For this review, take the finished solid that the model builds, in its own axes (mm). A direction names the side the tool comes from. Round coordinates to 2 decimals unless told otherwise and drop trailing zeros. Write each loop counter-clockwise with the first axis right and the second up, starting at its lowest first coordinate (ties: lowest second). Pieces come first, ordered by that corner, then holes. Notation, with made-up numbers: (26.5, -31.5) -> (81.5, -31.5) arc R20 ccw to (81.5, -21.5) -> close; hole circle Ø7 at (39.5, 58). An arc over 180 degrees is marked (long way). Answer in a Markdown table with one row per item.
from build123d import *

# Parameters (mm, degrees)
DODANIE_WYCI_GNI_CIE1_DEPTH = 130
SKORUPA1_T                  = -0.5
WYTNIJ_WYCI_GNI_CIE1_REACH  = 132
SZKIC2_W                    = 206
SZKIC2_H                    = 132
SZKIC4_R                    = 2
WYTNIJ_WYCI_GNI_CIE2_DEPTH  = 10
SZKIC5_R                    = 21.15
SZKIC5_R_2                  = 12.5
WYTNIJ_WYCI_GNI_CIE3_DEPTH  = 10
SZKIC6_R                    = 10
SZKIC6_R_2                  = 6
WYTNIJ_WYCI_GNI_CIE4_DEPTH  = 10
SZKIC7_R                    = 10.25
WYTNIJ_WYCI_GNI_CIE5_DEPTH  = 10


with BuildPart() as part:
    # Szkic1 → Dodanie-wyciągnięcie1 (new body)
    with BuildSketch(Plane.XY):
        Polygon((0, 403), (0, 185), (-30, 185), (-30, 0), (450, 0), (450, 403), align=None)
    extrude(amount=DODANIE_WYCI_GNI_CIE1_DEPTH)

    # Skorupa1
    skorupa1_openings = [part.faces().sort_by_distance(p)[0] for p in [
        (140, 196, 130),
    ]]
    offset(amount=SKORUPA1_T, openings=skorupa1_openings, kind=Kind.INTERSECTION)

    # Szkic2 → Wytnij-wyciągnięcie1 (cut, up to next)
    with BuildSketch(Plane(origin=(0, 0, 0), x_dir=(-1, 0, 0), z_dir=(0, 0, -1)), mode=Mode.PRIVATE) as wytnij_wyci_gni_cie1_sk1:
        with Locations((-329, 214)):
            Rectangle(SZKIC2_W, SZKIC2_H)
    wytnij_wyci_gni_cie1_tool1 = extrude(wytnij_wyci_gni_cie1_sk1.sketch, amount=-WYTNIJ_WYCI_GNI_CIE1_REACH, mode=Mode.PRIVATE) & part.part
    add(wytnij_wyci_gni_cie1_tool1.solids().sort_by_distance((329, 214, 0))[0], mode=Mode.SUBTRACT)

    # Szkic4 → Wytnij-wyciągnięcie2 (cut)
    with BuildSketch(Plane(origin=(0, 0, 0), x_dir=(-1, 0, 0), z_dir=(0, 0, -1))):
        with Locations((-114.4, 386.6)):
            Circle(SZKIC4_R)
        with Locations((-74.7, 365.2)):
            Circle(SZKIC4_R)
        with Locations((-74.7, 335.2)):
            Circle(SZKIC4_R)
        with Locations((-114.4, 356.6)):
            Circle(SZKIC4_R)
        with Locations((-74.7, 305.2)):
            Circle(SZKIC4_R)
        with Locations((-114.4, 326.6)):
            Circle(SZKIC4_R)
    extrude(amount=-WYTNIJ_WYCI_GNI_CIE2_DEPTH, mode=Mode.SUBTRACT)

    # Szkic5 → Wytnij-wyciągnięcie3 (cut)
    with BuildSketch(Plane(origin=(0, 403, 0), x_dir=(1, 0, 0), z_dir=(0, 1, 0))):
        with Locations((222.5, -77.9)):
            Circle(SZKIC5_R)
        with Locations((225.5, -23.7)):
            Circle(SZKIC5_R_2)
        with Locations((267.5, -23.7)):
            Circle(SZKIC5_R_2)
        with Locations((183.5, -23.7)):
            Circle(SZKIC5_R_2)
    extrude(amount=-WYTNIJ_WYCI_GNI_CIE3_DEPTH, mode=Mode.SUBTRACT)

    # Szkic6 → Wytnij-wyciągnięcie4 (cut)
    with BuildSketch(Plane.ZY.offset(30)):
        with Locations((74.5, 145)):
            Circle(SZKIC6_R)
        with Locations((74.5, 82)):
            Circle(SZKIC6_R)
        with Locations((13, 148)):
            Circle(SZKIC6_R_2)
        with Locations((13, 108)):
            Circle(SZKIC6_R_2)
        with Locations((13, 68)):
            Circle(SZKIC6_R_2)
    extrude(amount=-WYTNIJ_WYCI_GNI_CIE4_DEPTH, mode=Mode.SUBTRACT)

    # Szkic7 → Wytnij-wyciągnięcie5 (cut)
    with BuildSketch(Plane(origin=(0.5, 0, 0), x_dir=(0, 0, -1), z_dir=(1, 0, 0))):
        with Locations((-76, 224.23)):
            Circle(SZKIC7_R)
        with Locations((-76, 246.58)):
            Circle(SZKIC7_R)
        with BuildLine():
            Line((-87.5, 233.905), (-87.5, 236.905))
            ThreePointArc((-87.5, 236.905), (-85.25, 239.155), (-83, 236.905))
            Line((-83, 236.905), (-83, 233.905))
            ThreePointArc((-83, 233.905), (-85.25, 231.655), (-87.5, 233.905))
        make_face()
    extrude(amount=-WYTNIJ_WYCI_GNI_CIE5_DEPTH, mode=Mode.SUBTRACT)


solid = part.part
1) Mouldability with a two-part tool opening along X and no side actions: class faces 5 (the flat face through (228, 402.5, 50)), 6 (the flat face through (-30, 94, 64)), 7 (the cylindrical face through (237.423, 402.754, 19.945)), 8 (the cylindrical face through (0.25, 217.99, 84.13)) as pulls with the +X half, pulls with the -X half, needs draft (parallel to the pull), parting line crosses it, or undercut.
Solved:
| item | result |
|---|---|
| face 5 | undercut |
| face 6 | pulls with the -X half |
| face 7 | undercut |
| face 8 | needs draft |
2) Consider section A-A on x = 267.5. State the section outline as (y, z) points, then the cut area to 4 significant figures.
Solved:
| item | result |
|---|---|
| outline | (0, 0) -> (148, 0) -> (148, 0.5) -> (0.5, 0.5) -> (0.5, 130) -> (0, 130) -> close; (280, 0) -> (403, 0) -> (403, 11.2) -> (402.5, 11.2) -> (402.5, 0.5) -> (280, 0.5) -> close; (402.5, 36.2) -> (403, 36.2) -> (403, 130) -> (402.5, 130) -> close |
| area | 252.5 mm² |
3) For line 1 (X direction, y = 402.7, z = 23.7); line 2 (Y direction, x = -29.75, z = 13); line 3 (Y direction, x = 236.5, z = 101.5), list the stretches that pass through material, from the lowest coordinate up. Write a range as [from, to].
Solved:
| item | result |
|---|---|
| line 1 | [0, 171], [196, 213], [238, 255], [280, 450] |
| line 2 | [0, 62], [74, 102], [114, 142], [154, 185] |
| line 3 | [0, 0.5], [402.5, 403] |
4) Clearance check with flat-ended pins moving along their axes: pin 1 Ø2 at (x, y) = (64.5, 211.5) entering from +Z; pin 2 Ø20 at (x, z) = (267.5, 23.7) entering from -Y; pin 3 Ø24 at (x, z) = (-14, 75) entering from +Y. State where each tip first meets the part, or that it passes through.
Solved:
| item | result |
|---|---|
| pin 1 | z = 0.5 |
| pin 2 | y = 0 |
| pin 3 | y = 185 |
5) Consider section D-D on y = 82. State the section outline as (x, z) points.
Solved:
| item | result |
|---|---|
| outline | (-30, 0) -> (450, 0) -> (450, 130) -> (449.5, 130) -> (449.5, 0.5) -> (-29.5, 0.5) -> (-29.5, 64.5) -> (-30, 64.5) -> close; (-30, 84.5) -> (-29.5, 84.5) -> (-29.5, 130) -> (-30, 130) -> close |
6) Consider section B-B on y = 263. State the section outline as (x, z) points.
Solved:
| item | result |
|---|---|
| outline | (0, 0) -> (226, 0) -> (226, 0.5) -> (0.5, 0.5) -> (0.5, 130) -> (0, 130) -> close; (432, 0) -> (450, 0) -> (450, 130) -> (449.5, 130) -> (449.5, 0.5) -> (432, 0.5) -> close |
7) Consider section C-C on x = 35.5. State the section outline as (y, z) points, then the cut area to 3 significant figures.
Solved:
| item | result |
|---|---|
| outline | (0, 0) -> (403, 0) -> (403, 130) -> (402.5, 130) -> (402.5, 0.5) -> (0.5, 0.5) -> (0.5, 130) -> (0, 130) -> close |
| area | 331 mm² |
8) For faces 1 (the cylindrical face through (-29.75, 145.44, 64.51)), 2 (the flat face through (-15, 185, 64)), 3 (the flat face through (0.5, 295, 64)), 4 (the cylindrical face through (242.673, 402.754, 71.547)), list the 3-axis set-ups (+Z, -Z, +X, -X, +Y, -Y) from which the entire face can be reached by the end or side of a thin tool; tool diameter is ignored.
Solved:
| item | result |
|---|---|
| face 1 | -X |
| face 2 | +Z, -Z, -X, +Y |
| face 3 | +Z |
| face 4 | +Y |
